```python
from build123d import *

# Parameters (mm, degrees)
SKETCH1_W                       = 200
SKETCH1_H                       = 450
BOSS_EXTRUDE1_DEPTH             = 2.5
BOSS_EXTRUDE2_REACH             = 398.13
SKETCH2_R                       = 6.35
BOSS_EXTRUDE2_DIRECTION_2_REACH = 398.13
SKETCH3_R                       = 3.175
CUT_EXTRUDE1_DEPTH              = 493.483829684


with BuildPart() as part:
    # Sketch1 → Boss-Extrude1 (new, symmetric)
    with BuildSketch(Plane.XY):
        with Locations((100, 116.925373314)):
            Rectangle(SKETCH1_W, SKETCH1_H)
    extrude(amount=BOSS_EXTRUDE1_DEPTH, both=True)

    # Boss-Extrude2: up to this face of the body (flat: up to its plane)
    boss_extrude2_end = Plane(part.part.faces().sort_by_distance((100, 341.925373314, 0))[0])
    # Sketch2 → Boss-Extrude2 (add, up to the picked face)
    with BuildSketch(Plane(origin=(0, 0, 0), x_dir=(1, 0, 0), z_dir=(0, 1, 0)), mode=Mode.PRIVATE) as boss_extrude2_sk1:
        Circle(SKETCH2_R)
    boss_extrude2_tool1 = split(extrude(boss_extrude2_sk1.sketch, amount=BOSS_EXTRUDE2_REACH, mode=Mode.PRIVATE), bisect_by=boss_extrude2_end, keep=Keep.BOTH, mode=Mode.PRIVATE)
    add(boss_extrude2_tool1.solids().sort_by(Axis((0, 0, 0), (0, 1, 0)))[0])

    # Boss-Extrude2 direction 2: up to this face of the body (flat: up to its plane)
    boss_extrude2_direction_2_end = Plane(part.part.faces().sort_by_distance((100, -108.074626686, 0))[0])
    # Sketch2 → Boss-Extrude2 direction 2 (add, up to the picked face)
    with BuildSketch(Plane(origin=(0, 0, 0), x_dir=(1, 0, 0), z_dir=(0, 1, 0)), mode=Mode.PRIVATE) as boss_extrude2_direction_2_sk1:
        Circle(SKETCH2_R)
    boss_extrude2_direction_2_tool1 = split(extrude(boss_extrude2_direction_2_sk1.sketch, amount=-BOSS_EXTRUDE2_DIRECTION_2_REACH, mode=Mode.PRIVATE), bisect_by=boss_extrude2_direction_2_end, keep=Keep.BOTH, mode=Mode.PRIVATE)
    add(boss_extrude2_direction_2_tool1.solids().sort_by(Axis((0, 0, 0), (0, -1, 0)))[0])

    # Sketch3 → Cut-Extrude1 (cut, through all)
    with BuildSketch(Plane(origin=(0, 341.925373314, 0), x_dir=(1, 0, 0), z_dir=(0, 1, 0))):
        with Locations(Location((0, 0, 0), (0, 0, 180))):
            Circle(SKETCH3_R)
    extrude(amount=-CUT_EXTRUDE1_DEPTH, mode=Mode.SUBTRACT)


solid = part.part
```
Verification items for the finished model (mm, model axes). A direction names the side the tool comes from. Give positions to 0.01 mm unless a question says otherwise; leave off trailing zeros. Loops run counter-clockwise (first coordinate to the right, second up) from the corner with the lowest first, then second, coordinate; pieces in that order, holes last. Notation, with made-up numbers: M 85,-19.75 L 104,-19.75 A22 ccw 104,-10.75 Z; hole C 72,75.5 d1. An arc over 180 degrees is marked long. Return JSON: item names as keys, results as strings.
1) Material ranges on L1, parallel to X at y = 306.5, z = 0.5; L2, parallel to Z at x = 0, y = 33.5 (3 decimals); L3, parallel to X at y = 146, z = -0.25, recorded low to high. Write a range as [from, to].
Findings:
{"L1": "x = [-6.33, -3.14], [3.14, 200]", "L2": "z = [-6.35, -3.175], [3.175, 6.35]", "L3": "x = [-6.35, -3.17], [3.17, 200]"}
2) Gauge pin test, flat ends, axial feed: P1, Ø12, axis at x = 124, y = 251.5, coming from the -Z side; P2, Ø1.5, axis at x = 106.5, z = -5, coming from the +Y side. Record the tip position at first contact, or that the pin passes through.
Findings:
{"P1": "stops at z = -2.5", "P2": "passes through"}
3) Tool access check on faces 1 (the flat face through (72, -108.075, 0)), 2 (the flat face through (102, 120, -2.5)), 3 (the flat face through (102, 120, 2.5)). Record the directions out of +Z, -Z, +X, -X, +Y, -Y that give a thin tool (end or side, any length) a straight path to the whole face; none if there is none.
Findings:
{"face 1": "+Z, -Z, +X, -X, -Y", "face 2": "-Z, +X, +Y, -Y", "face 3": "+Z, +X, +Y, -Y"}
4) Section check A-A, the plane z = 0. Enter the section's corners in (x, y) (3 decimals).
Findings:
{"outline": "M -6.35,-108.075 L -3.175,-108.075 L -3.175,341.925 L -6.35,341.925 Z; M 3.175,-108.075 L 200,-108.075 L 200,341.925 L 3.175,341.925 Z"}
5) Section check B-B, the plane y = 251. Enter the section's corners in (x, z) (3 decimals).
Findings:
{"outline": "M 5.837,-2.5 L 200,-2.5 L 200,2.5 L 5.837,2.5 A6.35 ccw long Z; hole C 0,0 d6.35"}
6) Section check C-C, the plane x = 48. Enter the section's corners in (y, z).
Findings:
{"outline": "M -108.07,-2.5 L 341.93,-2.5 L 341.93,2.5 L -108.07,2.5 Z"}
